Here's how the part is built. I have some questions about the finished solid (model axes, mm). A direction names the side the tool comes from. Coordinates: 2 decimals unless noted, no trailing zeros. Loops run counter-clockwise (first coordinate to the right, second up) from the corner with the lowest first, then second, coordinate; pieces in that order, holes last. Notation, with made-up numbers: M -22,14 L -2,14 A34 ccw -2,50 Z; hole C 12.25,79.25 d11. An arc over 180 degrees is marked long. Use CSV: the item, a comma, the result in double quotes. Start each with the question number.
Q1. Please list where these lines run through material, in increasing order: probe 1 along Z at (x, y) = (50, 65.5); probe 2 along Y at (x, z) = (12, -24); probe 3 along Y at (x, z) = (34, 66.5). Write a range as [from, to].
Q2. If we section it at B-B (z = -1): Please give me the cut outline in (x, y).
Q3. If we mould it in two halves opening along X, with no side actions, what happens to faces 5 (the flat face through (-122.874, 146.593, -0.14)), 6 (the cylindrical face through (-54, 25, 0)), 7 (the flat face through (25, 63, 122))? For each: +X half, -X half, draft (parallel to the pull), parting line (faces both ways), or undercut.
Q4. If we section it at A-A (z = 24.5): Please give me the cut outline in (x, y).
Q5. If we section it at D-D (y = 64): Please give me the cut outline in (x, z).
Q6. For pin 1 Ø8 at (y, z) = (80, 3.5) entering from +X; pin 2 Ø3 at (x, y) = (-27, 61) entering from +Z; pin 3 Ø13.5 at (x, y) = (-83.5, 190.5) entering from +Z, each with a flat end and sliding along its axis, tell me the tip position at first contact or that it passes through.
Q7. If we section it at C-C (x = -39): Please give me the cut outline in (y, z).
Q8. Which directions (+Z, -Z, +X, -X, +Y, -Y) give clear straight access to the entire face, cutting with the end or side of a thin tool? Please do faces 1 (the flat face through (0, 37, -67)), 2 (the cylindrical face through (-104.58, 210.21, 35.64)), 3 (the flat face through (16, 22, -2)), 4 (the flat face through (0, 37, 65)).
from build123d import *

# Parameters (mm, degrees)
SKETCH8_R                 = 22.5
BOSS_EXTRUDE14_DEPTH      = 62
BOSS_EXTRUDE15_DEPTH      = 10
BOSS_EXTRUDE15_DEPTH_BACK = 10
SKETCH2_R                 = 12.5
SKETCH2_R_2               = 10
BOSS_EXTRUDE16_DEPTH      = 122
BOSS_EXTRUDE16_DEPTH_BACK = 122
SKETCH9_R                 = 12.5
CUT_EXTRUDE1_DEPTH        = 16


with BuildPart() as part:
    # Sketch8 → Boss-Extrude14 (new body)
    with BuildSketch(Plane.XY):
        with Locations((-88, 195)):
            Circle(SKETCH8_R)
    extrude(amount=BOSS_EXTRUDE14_DEPTH)

    # Sketch2 → Boss-Extrude15 (add, two sides: drawn at the far end of the back side and taken through both)
    with BuildSketch(Plane.XY.offset(-BOSS_EXTRUDE15_DEPTH_BACK)):
        with BuildLine():
            ThreePointArc((-56.190983138, 198.490909091), (-47.888697043, 171.070854158), (-30.246353585, 148.497970332))
            Line((-30.246353585, 148.497970332), (78, 85))
            Line((78, 85), (78, 75))
            Line((78, 75), (0, 75))
            Line((0, 75), (0, 0))
            Line((0, 0), (-44, 0))
            ThreePointArc((-44, 0), (-54.17497796, 2.164286227), (-62.588230747, 8.282414119))
            Line((-62.588230747, 8.282414119), (-116.254110736, 69.589269461))
            ThreePointArc((-116.254110736, 69.589269461), (-123.479967643, 81.392211935), (-126, 95))
            Line((-126, 95), (-119.660096955, 199.651694401))
            ThreePointArc((-119.660096955, 199.651694401), (-87.414850516, 226.994649554), (-56.190983138, 198.490909091))
        make_face()
        with Locations((-88, 95)):
            Circle(SKETCH2_R, mode=Mode.SUBTRACT)
        with Locations((-44, 25)):
            Circle(SKETCH2_R_2, mode=Mode.SUBTRACT)
    extrude(amount=BOSS_EXTRUDE15_DEPTH + BOSS_EXTRUDE15_DEPTH_BACK)

    # Sketch3 → Boss-Extrude16 (add, two sides: drawn at the far end of the back side and taken through both)
    with BuildSketch(Plane.XY.offset(-BOSS_EXTRUDE16_DEPTH_BACK)):
        with BuildLine():
            Line((0, 0), (0, 75))
            Line((0, 75), (78, 75))
            Line((78, 75), (88, 75))
            Line((88, 75), (88, 59))
            Line((88, 59), (32, 59))
            ThreePointArc((32, 59), (20.686291501, 54.313708499), (16, 43))
            Line((16, 43), (16, 0))
            Line((16, 0), (0, 0))
        make_face()
    extrude(amount=BOSS_EXTRUDE16_DEPTH + BOSS_EXTRUDE16_DEPTH_BACK)

    # Sketch9 → Cut-Extrude1 (cut)
    with BuildSketch(Plane(origin=(0, 75, 0), x_dir=(1, 0, 0), z_dir=(0, 1, 0))):
        with Locations(Location((50, -84, 0), (0, 0, 180))):
            Circle(SKETCH9_R)
        with Locations(Location((50, 84, 0), (0, 0, 180))):
            Circle(SKETCH9_R)
    extrude(amount=-CUT_EXTRUDE1_DEPTH, mode=Mode.SUBTRACT)


solid = part.part
Results below:
1,probe 1,"[-122, -96.5], [-71.5, 71.5], [96.5, 122]"
1,probe 2,"[0, 75]"
1,probe 3,"[59, 75]"
2,outline,"M -126,95 A38 ccw -116.25,69.59 L -62.59,8.28 A25 ccw -44,0 L 16,0 L 16,43 A16 cw 32,59 L 88,59 L 88,75 L 78,75 L 78,85 L -30.25,148.5 A78 cw -56.19,198.49 A32 ccw -119.66,199.65 Z; hole C -88,95 d25; hole C -44,25 d20"
3,face 5,"-X half"
3,face 6,"undercut"
3,face 7,"draft"
4,outline,"C -88,195 d45; M 0,0 L 16,0 L 16,43 A16 cw 32,59 L 88,59 L 88,75 L 0,75 Z"
5,outline,"M -111.36,-10 L 0,-10 L 0,-122 L 88,-122 L 88,122 L 0,122 L 0,10 L -111.36,10 Z; hole C 50,-84 d25; hole C 50,84 d25"
6,pin 1,"x = 78"
6,pin 2,"z = 10"
6,pin 3,"z = 62"
7,outline,"M 0,-10 L 16.34,-10 L 16.34,10 L 0,10 Z; M 33.66,-10 L 157.58,-10 L 157.58,10 L 33.66,10 Z"
8,face 1,"-Z, -X, +Y, -Y"
8,face 2,"+Z"
8,face 3,"+Z, -Z, +X, -Y"
8,face 4,"+Z, -X, +Y, -Y"
